```python
from build123d import *

# Parameters (mm, degrees)
BOX001_W     = 2.4
BOX001_H     = 24
BOX001_DEPTH = 22
BOX002_W     = 2.4
BOX002_H     = 24
BOX002_DEPTH = 22
BOX003_W     = 2.4
BOX003_H     = 24
BOX003_DEPTH = 22
BOX_W        = 2.4
BOX_H        = 24
BOX_DEPTH    = 22
BOX004_W     = 33
BOX004_H     = 30
BOX004_DEPTH = 10


with BuildPart() as cube001:
    # Box001 → Box001 (new body)
    with BuildSketch(Plane(origin=(8.1, 3, 0), x_dir=(1, 0, 0), z_dir=(0, 0, 1))):
        with Locations((1.2, 12)):
            Rectangle(BOX001_W, BOX001_H)
    extrude(amount=BOX001_DEPTH)


with BuildPart() as cube002:
    # Box002 → Box002 (new body)
    with BuildSketch(Plane(origin=(13.7, 3, 0), x_dir=(1, 0, 0), z_dir=(0, 0, 1))):
        with Locations((1.2, 12)):
            Rectangle(BOX002_W, BOX002_H)
    extrude(amount=BOX002_DEPTH)


with BuildPart() as cube003:
    # Box003 → Box003 (new body)
    with BuildSketch(Plane(origin=(19.3, 3, 0), x_dir=(1, 0, 0), z_dir=(0, 0, 1))):
        with Locations((1.2, 12)):
            Rectangle(BOX003_W, BOX003_H)
    extrude(amount=BOX003_DEPTH)


with BuildPart() as fusion:
    # Box → Box (new body)
    with BuildSketch(Plane(origin=(2.5, 3, 0), x_dir=(1, 0, 0), z_dir=(0, 0, 1))):
        with Locations((1.2, 12)):
            Rectangle(BOX_W, BOX_H)
    extrude(amount=BOX_DEPTH)

    # Fusion: union Cube001, Cube002, Cube003
    add(cube001.part)
    add(cube002.part)
    add(cube003.part)


with BuildPart() as fusion_1:
    # Fusion placement: moved
    add(fusion.part.moved(Location((0, 0, 3))))


with BuildPart() as cut:
    # Box004 → Box004 (new body)
    with BuildSketch(Plane(origin=(-4.5, 0, 0), x_dir=(1, 0, 0), z_dir=(0, 0, 1))):
        with Locations((16.5, 15)):
            Rectangle(BOX004_W, BOX004_H)
    extrude(amount=BOX004_DEPTH)

    # Cut: cut Fusion
    add(fusion_1.part, mode=Mode.SUBTRACT)


solid = cut.part
```
Read the model definition and answer for the solid it produces. Units are mm, in the model's axes. A direction names the side the tool comes from. Give positions to 0.01 mm unless a question says otherwise; leave off trailing zeros. Order: outer loops, then holes, each group sorted by start corner. A loop starts at its lowest first (then second) coordinate and runs counter-clockwise, first axis right, second up. Notation, with made-up numbers: (-1, 24) -> (28, 24) arc R21 ccw to (28, 34) -> close; hole circle Ø8 at (71.5, 26.25). An arc over 180 degrees is marked (long way). One line per item, written item: value. Start each with the question number.
(1) Straight lines are drawn through the part: L1, parallel to X at y = 14.5, z = 9.25; L2, parallel to Z at x = 20.5, y = 22.75. For each, find the intervals that lie inside material, in ascending order.
(2) A flat-ended cylindrical pin translates along its axis: P1, Ø0.7, axis at x = 20, y = 14, coming from the +Z side. Find the tip coordinate at first contact, or state that the pin passes through.
(3) A tool of negligible diameter and unlimited length cuts with its end or side. For faces 1 (the flat face through (12, 0, 5)), 2 (the flat face through (20, 27, 6)), from which of +Z, -Z, +X, -X, +Y, -Y can it reach the whole face along a straight path? Write none if from no direction.
(4) The part is cut by section A-A (z = 4). Determine the outline of the cut face in (x, y), and give its area (3 significant figures).
(5) For a pull along X with two mould halves and no side action, classify faces 3 (the flat face through (15, 27, 6)), 4 (the flat face through (12, 30, 5)), 5 (the flat face through (28.5, 15, 5)) as released by +X, released by -X, zero draft, split by the parting line, or undercut.
(6) The part is cut by section C-C (y = 24). Determine the outline of the cut face in (x, z).
(7) The part is cut by section B-B (x = 20). Determine the outline of the cut face in (y, z), and give its area (3 significant figures).
Taken from the geometry:
1. L1: -4.5 to 2.5, 4.9 to 8.1, 10.5 to 13.7, 16.1 to 19.3, 21.7 to 28.5
1. L2: 0 to 3
2. P1: z = 3
3. face 1: +Z, -Z, +X, -X, -Y
3. face 2: +Z
4. outline: (-4.5, 0) -> (28.5, 0) -> (28.5, 30) -> (-4.5, 30) -> close; hole (2.5, 3) -> (4.9, 3) -> (4.9, 27) -> (2.5, 27) -> close; hole (8.1, 3) -> (10.5, 3) -> (10.5, 27) -> (8.1, 27) -> close; hole (13.7, 3) -> (16.1, 3) -> (16.1, 27) -> (13.7, 27) -> close; hole (19.3, 3) -> (21.7, 3) -> (21.7, 27) -> (19.3, 27) -> close
4. area: 760 mm^2
5. face 3: undercut
5. face 4: zero draft
5. face 5: released by +X
6. outline: (-4.5, 0) -> (28.5, 0) -> (28.5, 10) -> (21.7, 10) -> (21.7, 3) -> (19.3, 3) -> (19.3, 10) -> (16.1, 10) -> (16.1, 3) -> (13.7, 3) -> (13.7, 10) -> (10.5, 10) -> (10.5, 3) -> (8.1, 3) -> (8.1, 10) -> (4.9, 10) -> (4.9, 3) -> (2.5, 3) -> (2.5, 10) -> (-4.5, 10) -> close
7. outline: (0, 0) -> (30, 0) -> (30, 10) -> (27, 10) -> (27, 3) -> (3, 3) -> (3, 10) -> (0, 10) -> close
7. area: 132 mm^2
